```python
from build123d import *

# Parameters (mm, degrees)
SKETCH_1_R      = 3
EXTRUDE_1_DEPTH = 3
FILLET_1_R      = 5


with BuildPart() as part:
    # ｽｹｯﾁ1 → ﾎﾞｽ - 押し出し1 (new body)
    with BuildSketch(Plane.XY):
        Polygon((1.518334957, 53.544180062), (-51.352653687, -5), (5.336736491, -5), align=None)
        with Locations((-2.700997506, 41.412010486)):
            Circle(SKETCH_1_R, mode=Mode.SUBTRACT)
        with Locations((-40.1, 0)):
            Circle(SKETCH_1_R, mode=Mode.SUBTRACT)
        Circle(SKETCH_1_R, mode=Mode.SUBTRACT)
    extrude(amount=EXTRUDE_1_DEPTH)

    # ﾌｨﾚｯﾄ1
    fillet_1_edges = [part.edges().sort_by_distance(p)[0] for p in [
        (5.336736491, -5, 1.5),
        (-51.352653687, -5, 1.5),
        (1.518334957, 53.544180062, 1.5),
    ]]
    fillet(fillet_1_edges, radius=FILLET_1_R)


solid = part.part
```
Can you work these out from the model? Positions are in its coordinate system, mm. Coordinates: 2 decimals unless noted, no trailing zeros. Loops run counter-clockwise (first coordinate to the right, second up) from the corner with the lowest first, then second, coordinate; pieces in that order, holes last. Notation, with made-up numbers: (0.5, 15.25) - (33.5, 15.25) arc R24 cw to (33.5, 51.25) - close; hole circle Ø3 at (19, 41.25). An arc over 180 degrees is marked (long way). Use a Markdown table: item, result.
Item 1: We'd pull the mould along Y, two halves only. Please class faces 1 (the face through (-43.1, 0.1, 1.5)), 2 (the face through (-44.7, -1.96, 1.52)), 3 (the face through (-15, 15, 0)): released by +Y, released by -Y, zero draft, split by the parting line, or undercut.
Numbers:
| item | result |
|---|---|
| face 1 | undercut |
| face 2 | split by the parting line |
| face 3 | zero draft |
Item 2: I want a section at C-C on y = 13. Please give me the cut outline in (x, z).
Numbers:
| item | result |
|---|---|
| outline | (-35.1, 0) - (4.16, 0) - (4.16, 3) - (-35.1, 3) - close |
Item 3: I want a section at A-A on z = 0.95. Please give me the cut outline in (x, y), and give its area (3 significant figures).
Numbers:
| item | result |
|---|---|
| outline | (-43.81, 3.35) arc R5 ccw to (-40.1, -5) - (0, -5) arc R5 ccw to (4.99, 0.33) - (2.29, 41.74) arc R5 ccw to (-6.41, 44.76) - close; hole circle Ø6 at (-40.1, 0); hole circle Ø6 at (-2.7, 41.41); hole circle Ø6 at (0, 0) |
| area | 1,510 mm2 |
Item 4: If I drill on probe 1 along Y at (x, z) = (-1, 1.95); probe 2 along Y at (x, z) = (0, 0.3); probe 3 along X at (y, z) = (-0.5, 2.15), over which ranges is the centre line in solid material (lowest first)? Write a range as from..to.
Numbers:
| item | result |
|---|---|
| probe 1 | y = -5..-2.83, 2.83..38.94, 43.88..46.11 |
| probe 2 | y = -5..-3, 3..40.11, 42.72..45.62 |
| probe 3 | x = -45.07..-43.06, -37.14..-2.96, 2.96..4.97 |
Item 5: I want a section at B-B on x = -27.5. Please give me the cut outline in (y, z), and give its area (3 significant figures).
Numbers:
| item | result |
|---|---|
| outline | (-5, 0) - (21.41, 0) - (21.41, 3) - (-5, 3) - close |
| area | 79.2 mm2 |
